Can you work these out from the model? Positions are in its coordinate system, mm. A direction names the side the tool comes from. Give positions to 0.01 mm unless a question says otherwise; leave off trailing zeros. Loops run counter-clockwise (first coordinate to the right, second up) from the corner with the lowest first, then second, coordinate; pieces in that order, holes last. Notation, with made-up numbers: (70, -33.5) - (76, -33.5) arc R15 cw to (76, -24.5) - close; hole circle Ø8 at (76.5, 48). An arc over 180 degrees is marked (long way). Answer as a JSON object with one key per item and string values.
Autodesk Inventor part; units mm, degrees
ref_plane "YZ Plane" through (0, 0, 0) normal (1, 0, 0) x (0, 1, 0)
ref_plane "XZ Plane" through (0, 0, 0) normal (0, 1, 0) x (-1, 0, 0)
ref_plane "XY Plane" through (0, 0, 0) normal (0, 0, 1) x (1, 0, 0)
sketch "Esboço1" plane through (0, 0, 0) normal (0, 1, 0) x (-1, 0, 0)
  line L0 (11.8731, -18.4543) -> (11.8731, 18.5457)
  line L1 (11.8731, 18.5457) -> (19.8731, 18.5457)
  line L2 (19.8731, 18.5457) -> (19.8731, -18.4543)
  line L3 (19.8731, -18.4543) -> (11.8731, -18.4543)
  line L4 (11.8731, -18.4543) -> (11.8731, 18.5457)
  circle A0 centre (15.8731, 12.5457) radius 1.5
  circle A1 centre (15.8731, -12.4543) radius 1.5
  line L5 (14.1231, -18.4543) -> (14.1231, 18.5457)
  point P0 (15.8731, 18.5457)
  point P1 (15.8731, -18.4543)
  dimension "d2" = 8
  dimension "d3" = 3
  dimension "d5" = 6
  dimension "d6" = 6
  dimension "d8" = 4
  dimension "d9" = 2.25
  dimension "d10" = 3
extrude "Extrusão1" add sketch "Esboço1" along normal blind 2.5 contours L5 L1 L2 L3
extrude "Extrusão2" add sketch "Esboço1" along normal blind 15.5 contours L0 L1 L5 L3
properties part number "pecinha_empunhadura"
1) I need wall thicknesses on L1, parallel to X at y = 5.5, z = -7; L2, parallel to Y at x = -18, z = 3; L3, parallel to X at y = 2, z = -12. Which ranges of each line are inside material? Lowest first, please.
Check sheet entries:
{"L1": "-14.12 to -11.87", "L2": "0 to 2.5", "L3": "-19.87 to -17.3, -14.44 to -11.87"}
2) If we mould it in two halves opening along X, with no side actions, what happens to faces 1 (the flat face through (-16, 0, 0)), 2 (the cylindrical face through (-14.683, 1.232, 13.458)), 3 (the flat face through (-19.873, 1, 0))? For each: released by +X, released by -X, zero draft, split by the parting line, or undercut.
Check sheet entries:
{"face 1": "zero draft", "face 2": "undercut", "face 3": "released by -X"}
3) Which directions (+Z, -Z, +X, -X, +Y, -Y) give clear straight access to the entire face, cutting with the end or side of a thin tool? Please do faces 4 (the cylindrical face through (-14.375, 1.232, -12.52)), 5 (the flat face through (-14.123, 9, 0)).
Check sheet entries:
{"face 4": "+Y, -Y", "face 5": "+Z, -Z, -X, +Y"}
4) Imagine slicing it at D-D on z = -13.5. Write out the boundary of the cut face in (x, y), and give its area (3 significant figures).
Check sheet entries:
{"outline": "(-19.87, 0) - (-16.95, 0) - (-16.95, 2.5) - (-19.87, 2.5) - close; (-14.8, 0) - (-11.87, 0) - (-11.87, 15.5) - (-14.12, 15.5) - (-14.12, 2.5) - (-14.8, 2.5) - close", "area": "43.9 mm2"}
5) Imagine slicing it at A-A on x = -17. Write out the boundary of the cut face in (y, z), and give its area (3 significant figures).
Check sheet entries:
{"outline": "(0, -18.45) - (2.5, -18.45) - (2.5, -13.44) - (0, -13.44) - close; (0, -11.46) - (2.5, -11.46) - (2.5, 11.56) - (0, 11.56) - close; (0, 13.54) - (2.5, 13.54) - (2.5, 18.55) - (0, 18.55) - close", "area": "82.6 mm2"}
6) I'm going to push flat-ended pins straight in: P1, Ø3, axis at x = -18.5, z = 0.5, coming from the +Y side; P2, Ø1.5, axis at y = 9.5, z = 3, coming from the -X side. Where does each tip first touch, or does it pass through?
Check sheet entries:
{"P1": "y = 2.5", "P2": "x = -14.12"}
7) Imagine slicing it at C-C on y = 1.5. Write out the boundary of the cut face in (x, z), and give its area (3 significant figures).
Check sheet entries:
{"outline": "(-19.87, -18.45) - (-11.87, -18.45) - (-11.87, 18.55) - (-19.87, 18.55) - close; hole circle Ø3 at (-15.87, -12.45); hole circle Ø3 at (-15.87, 12.55)", "area": "282 mm2"}
8) Imagine slicing it at B-B on z = -9. Write out the boundary of the cut face in (x, y).
Check sheet entries:
{"outline": "(-19.87, 0) - (-11.87, 0) - (-11.87, 15.5) - (-14.12, 15.5) - (-14.12, 2.5) - (-19.87, 2.5) - close"}
